The model under review builds one solid part; all positions refer to its coordinate system, in mm. Face numbers are marked on the shaded views. A direction names the side the tool comes from. Coordinates: 2 decimals unless noted, no trailing zeros. Order: outer loops, then holes, each group sorted by start corner. A loop starts at its lowest first (then second) coordinate and runs counter-clockwise, first axis right, second up. Notation, with made-up numbers: (75.25, -32.75) -> (119.25, -32.75) arc R7 cw to (119.25, -24.75) -> close; hole circle Ø10 at (73.25, -26). An arc over 180 degrees is marked (long way). Put each result on its own line as item: value.
from build123d import *

# Parameters (mm, degrees)
SKETCH1_W            = 30
SKETCH1_H            = 13
BOTTOMPLATEAU_DEPTH  = 7.12
SKETCH3_R            = 1.5
SCREWSOCKETS_DEPTH   = 1.5
SKETCH4_W            = 30
SKETCH4_H            = 8.4
TOPPLATEAU_DEPTH     = 4.3
SKETCH5_W            = 7.5
SKETCH5_H            = 7.2
SKETCH5_W_2          = 16.3
SENSORSOCKETS_DEPTH  = 2
EXTRUDEDSLANTS_DEPTH = 4
F_45SLANTS_DEPTH     = 7.5
CONNECTION_W         = 10
CONNECTION_H         = 6.12
BOSS_EXTRUDE6_DEPTH  = 10


with BuildPart() as part:
    # Sketch1 → BottomPlateau (new body)
    with BuildSketch(Plane(origin=(0, 0, 0), x_dir=(1, 0, 0), z_dir=(0, 1, 0))):
        Rectangle(SKETCH1_W, SKETCH1_H)
    extrude(amount=BOTTOMPLATEAU_DEPTH)

    # Sketch3 → ScrewSockets (add)
    with BuildSketch(Plane.XZ):
        with BuildLine():
            Line((-18.75, 3.75), (-15, 3.75))
            Line((-15, 3.75), (-15, -3.75))
            Line((-15, -3.75), (-18.75, -3.75))
            ThreePointArc((-18.75, -3.75), (-22.5, 0), (-18.75, 3.75))
        make_face()
        with Locations((-18.75, 0)):
            Circle(SKETCH3_R, mode=Mode.SUBTRACT)
        with BuildLine():
            Line((18.75, 3.75), (15, 3.75))
            Line((15, 3.75), (15, -3.75))
            Line((15, -3.75), (18.75, -3.75))
            ThreePointArc((18.75, -3.75), (22.5, 0), (18.75, 3.75))
        make_face()
        with Locations((18.75, 0)):
            Circle(SKETCH3_R, mode=Mode.SUBTRACT)
    extrude(amount=-SCREWSOCKETS_DEPTH)

    # Sketch4 → TopPlateau (add)
    with BuildSketch(Plane(origin=(0, 7.12, 0), x_dir=(1, 0, 0), z_dir=(0, 1, 0))):
        Rectangle(SKETCH4_W, SKETCH4_H)
    extrude(amount=TOPPLATEAU_DEPTH)

    # Sketch5 → SensorSockets (add)
    with BuildSketch(Plane(origin=(0, 11.42, 0), x_dir=(1, 0, 0), z_dir=(0, 1, 0))):
        with Locations((-10.2, 0)):
            Rectangle(SKETCH5_W, SKETCH5_H)
        with Locations((5.8, 0)):
            Rectangle(SKETCH5_W_2, SKETCH5_H)
    extrude(amount=SENSORSOCKETS_DEPTH)

    # Sketch6 → ExtrudedSlants (add)
    with BuildSketch(Plane(origin=(0, 1.5, 0), x_dir=(1, 0, 0), z_dir=(0, 1, 0))):
        with BuildLine():
            Line((-15, -3.75), (-15, 0))
            ThreePointArc((-15, 0), (-16.098349571, -2.651650429), (-18.75, -3.75))
            Line((-18.75, -3.75), (-15, -3.75))
        make_face()
        with BuildLine():
            Line((-15, 3.75), (-18.75, 3.75))
            ThreePointArc((-18.75, 3.75), (-16.098349571, 2.651650429), (-15, 0))
            Line((-15, 0), (-15, 3.75))
        make_face()
        with BuildLine():
            ThreePointArc((15, 6e-09), (16.098349573, 2.651650432), (18.75, 3.75))
            Line((18.75, 3.75), (15, 3.75))
            Line((15, 3.75), (15, 6e-09))
        make_face()
        with BuildLine():
            ThreePointArc((18.75, -3.75), (16.098349568, -2.651650427), (15, 6e-09))
            Line((15, 6e-09), (15, -3.75))
            Line((15, -3.75), (18.75, -3.75))
        make_face()
    extrude(amount=EXTRUDEDSLANTS_DEPTH)

    # Sketch7 → 45Slants (cut)
    with BuildSketch(Plane.XY.offset(3.75)):
        Polygon((-15, 5.5), (-18.75, 1.75), (-18.75, 5.5), align=None)
        Polygon((15, 5.5), (18.75, 1.75), (18.75, 5.5), align=None)
    extrude(amount=-F_45SLANTS_DEPTH, mode=Mode.SUBTRACT)

    # Connection → Boss-Extrude6 (add)
    with BuildSketch(Plane.XY.offset(4.2)):
        with Locations((0, 6.06)):
            Rectangle(CONNECTION_W, CONNECTION_H)
    extrude(amount=BOSS_EXTRUDE6_DEPTH)


solid = part.part
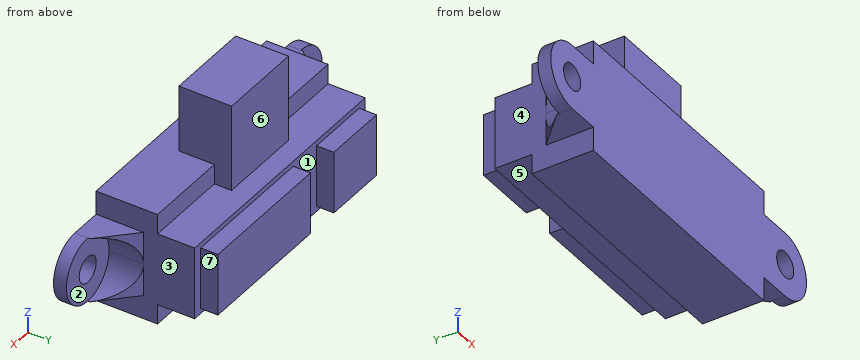
Item 1: Consider section C-C on y = 6. Write out the cut boundary in (x, z), and give its area (3 significant figures).
Answers below:
outline: (-15, -6.5) -> (15, -6.5) -> (15, 6.5) -> (5, 6.5) -> (5, 14.2) -> (-5, 14.2) -> (-5, 6.5) -> (-15, 6.5) -> close
area: 467 mm^2
Item 2: For pin 1 Ø1.6 at (x, y) = (-9.5, 12.5) entering from +Z; pin 2 Ø1.9 at (x, y) = (17.5, 1.5) entering from -Z; pin 3 Ø1 at (y, z) = (10, 3.5) entering from +X, all flat-tipped, find the tip position at first contact; note any pin that passes through.
Answers below:
pin 1: z = 3.6
pin 2: z = -3.75
pin 3: x = 15
Item 3: Consider section D-D on z = 9.5. Write out the cut boundary in (x, y).
Answers below:
outline: (-5, 3) -> (5, 3) -> (5, 9.12) -> (-5, 9.12) -> close
Item 4: For line 1 (Z direction, x = -18.75, y = 1); line 2 (Z direction, x = 12.5, y = 12.5), list the stretches that pass through material, from the lowest coordinate up. Write a range as from..to.
Answers below:
line 1: -3.75..-1.5, 1.5..3.75
line 2: -3.6..3.6
Item 5: Consider section A-A on x = 3. Write out the cut boundary in (y, z), and give its area (3 significant figures).
Answers below:
outline: (0, -6.5) -> (7.12, -6.5) -> (7.12, -4.2) -> (11.42, -4.2) -> (11.42, -3.6) -> (13.42, -3.6) -> (13.42, 3.6) -> (11.42, 3.6) -> (11.42, 4.2) -> (9.12, 4.2) -> (9.12, 14.2) -> (3, 14.2) -> (3, 6.5) -> (0, 6.5) -> close
area: 195 mm^2
Item 6: For the marked faces 4, 5, 6 and 7, list the 3-axis set-ups (+Z, -Z, +X, -X, +Y, -Y) from which the entire face can be reached by the end or side of a thin tool; tool diameter is ignored.
Answers below:
face 4: -X, +Y
face 5: -Z, +X, -X, +Y
face 6: +Z, +X, -X, +Y
face 7: +Z, -Z, +X, +Y
Item 7: Mouldability with a two-part tool opening along X and no side actions: class the marked faces 1, 2 and 3 as +X half, -X half, draft (parallel to the pull), parting line (faces both ways), or undercut.
Answers below:
face 1: undercut
face 2: draft
face 3: +X half
Item 8: Consider section B-B on z = -0.75. Write out the cut boundary in (x, y), and give its area (3 significant figures).
Answers below:
outline: (-22.42, 0) -> (-20.05, 0) -> (-20.05, 1.5) -> (-22.42, 1.5) -> close; (-17.45, 0) -> (17.45, 0) -> (17.45, 1.5) -> (15.08, 1.5) -> (15.08, 5.42) -> (15, 5.5) -> (15, 11.42) -> (13.95, 11.42) -> (13.95, 13.42) -> (-2.35, 13.42) -> (-2.35, 11.42) -> (-6.45, 11.42) -> (-6.45, 13.42) -> (-13.95, 13.42) -> (-13.95, 11.42) -> (-15, 11.42) -> (-15, 5.5) -> (-15.08, 5.42) -> (-15.08, 1.5) -> (-17.45, 1.5) -> close; (20.05, 0) -> (22.42, 0) -> (22.42, 1.5) -> (20.05, 1.5) -> close
area: 405 mm^2
